```python
from build123d import *
from build123d.topology import SkipClean

# Parameters (mm, degrees)
BOSS_EXTRUDE1_DEPTH = 5
BOSS_EXTRUDE3_DEPTH = 5
BOSS_EXTRUDE4_DEPTH = 5.043608808
CIRPATTERN1_COUNT   = 3


with BuildPart() as part:
    # Sketch1 → Boss-Extrude1 (new body)
    with BuildSketch(Plane.XY):
        with BuildLine():
            ThreePointArc((0, 5), (-1.701397984, 4.701621518), (-3.199731749, 3.84209796))
            ThreePointArc((-3.199731749, 3.84209796), (-3.824264635, 3.221024682), (-4.330127019, 2.5))
            Line((-4.330127019, 2.5), (-2.165063509, 1.25))
            ThreePointArc((-2.165063509, 1.25), (-1.25, 2.165063509), (0, 2.5))
            Line((0, 2.5), (0, 5))
        make_face()
        with BuildLine():
            ThreePointArc((0, 7.5), (-1.894259298, 7.256843784), (-3.665691684, 6.54314179))
            Line((-3.665691684, 6.54314179), (-3.199731749, 3.84209796))
            ThreePointArc((-3.199731749, 3.84209796), (-1.701397984, 4.701621518), (0, 5))
            Line((0, 5), (0, 7.5))
        make_face()
        with BuildLine():
            Line((-3.199731749, 3.84209796), (-3.665691684, 6.54314179))
            ThreePointArc((-3.665691684, 6.54314179), (-5.268898566, 5.337481419), (-6.495190528, 3.75))
            Line((-6.495190528, 3.75), (-4.330127019, 2.5))
            ThreePointArc((-4.330127019, 2.5), (-3.824264635, 3.221024682), (-3.199731749, 3.84209796))
        make_face()
        with BuildLine():
            ThreePointArc((0, 14.1), (-3.800809124, 15.48736773), (-5.814119968, 18.997))
            Line((-5.814119968, 18.997), (-3.665691684, 6.54314179))
            ThreePointArc((-3.665691684, 6.54314179), (-1.894259298, 7.256843784), (0, 7.5))
            Line((0, 7.5), (0, 14.1))
        make_face()
        with BuildLine():
            ThreePointArc((0, 25.9), (-4.51263227, 23.800809124), (-5.814119968, 18.997))
            ThreePointArc((-5.814119968, 18.997), (-3.800809124, 15.48736773), (0, 14.1))
            Line((0, 14.1), (0, 16))
            ThreePointArc((0, 16), (-4, 20), (0, 24))
            Line((0, 24), (0, 25.9))
        make_face()
        with BuildLine():
            ThreePointArc((0, 2.5), (-1.25, 2.165063509), (-2.165063509, 1.25))
            Line((-2.165063509, 1.25), (0, 0))
            Line((0, 0), (0, 2.5))
        make_face()
    extrude(amount=BOSS_EXTRUDE1_DEPTH)

    # Sketch2 → Boss-Extrude3 (add)
    with BuildSketch(Plane.XY.offset(5)):
        with BuildLine():
            ThreePointArc((0, 16), (-4, 20), (0, 24))
            Line((0, 24), (0, 25.9))
            ThreePointArc((0, 25.9), (-4.51263227, 23.800809124), (-5.814119968, 18.997))
            Line((-5.814119968, 18.997), (-3.199731749, 3.84209796))
            ThreePointArc((-3.199731749, 3.84209796), (-3.824264635, 3.221024682), (-4.330127019, 2.5))
            Line((-4.330127019, 2.5), (0, 0))
            Line((0, 0), (0, 16))
        make_face()
    extrude(amount=BOSS_EXTRUDE3_DEPTH)

    # Sketch4 → Boss-Extrude4 (add)
    with BuildSketch(Plane.XY.offset(10)):
        with BuildLine():
            ThreePointArc((0, 2.5), (-1.25, 2.165063509), (-2.165063509, 1.25))
            Line((-2.165063509, 1.25), (0, 0))
            Line((0, 0), (0, 2.5))
        make_face()
        with BuildLine():
            Line((-4.330127019, 2.5), (-2.165063509, 1.25))
            ThreePointArc((-2.165063509, 1.25), (-1.25, 2.165063509), (0, 2.5))
            Line((0, 2.5), (0, 5))
            ThreePointArc((0, 5), (-1.701397984, 4.701621518), (-3.199731749, 3.84209796))
            ThreePointArc((-3.199731749, 3.84209796), (-3.824264635, 3.221024682), (-4.330127019, 2.5))
        make_face()
    extrude(amount=BOSS_EXTRUDE4_DEPTH)

    # Mirror1: part across plane


with BuildPart() as part_1:
    with SkipClean():  # the faces are left unmerged after this step: merging them gives an invalid solid
        add(part.part)
        add(part.part.mirror(Plane(origin=(0, 0, 0), x_dir=(0, 0, 1), z_dir=(1, 0, 0))))


with BuildPart() as cirpattern1_1:
    # CirPattern1: pattern copy
    add(part_1.part.rotate(Axis((0, 0, 0), (0, 0, 1)), 1 * 360 / CIRPATTERN1_COUNT))


with BuildPart() as cirpattern1_2:
    # CirPattern1: pattern copy
    add(part_1.part.rotate(Axis((0, 0, 0), (0, 0, 1)), 2 * 360 / CIRPATTERN1_COUNT))


with BuildPart() as part_2:
    add(part_1.part)

    # Combine1: union CirPattern1_2, CirPattern1_1
    add(cirpattern1_2.part)
    add(cirpattern1_1.part)

    # Sketch8 → M5 Tapped Hole1 (revolve, cut)
    with SkipClean():  # the faces are left unmerged after this step: merging them gives an invalid solid
        with BuildSketch(Plane(origin=(0, 0, 15.043608808), x_dir=(0, -1, 0), z_dir=(1, 0, 0))):
            Polygon((0, 0), (0, 15.043608808), (2.525, 15.043608808), (2.1, 14.618608808), (2.1, 0.425), (2.525, 0), align=None)
        revolve(axis=Axis((0, 0, 21.393608808), (0, 0, -1)), mode=Mode.SUBTRACT)


solid = part_2.part
```
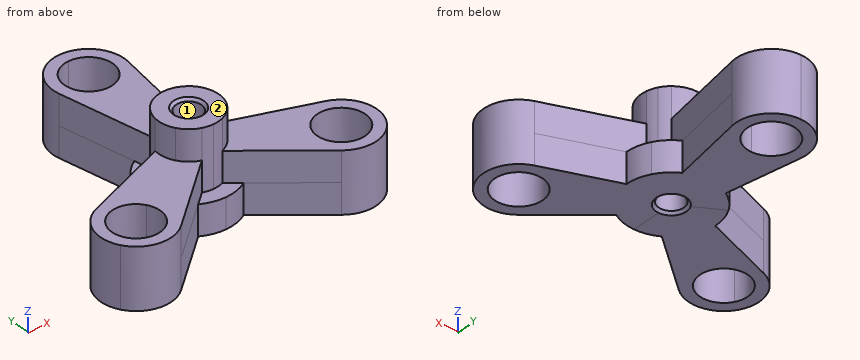
The listing builds one solid part. Answer for the finished solid, in the listing's coordinates (mm). Face numbers are marked on the shaded views. Round coordinates to 2 decimals unless told otherwise and drop trailing zeros. Write each loop counter-clockwise with the first axis right and the second up, starting at its lowest first coordinate (ties: lowest second). Pieces come first, ordered by that corner, then holes. Notation, with made-up numbers: (-25.75, -17.75) -> (28.25, -17.75) arc R7 ccw to (28.25, -12.75) -> close; hole circle Ø11 at (31, -5.5). An arc over 180 degrees is marked (long way). Use CSV: the item, a comma, the result in double quotes. Start each with the question number.
(1) Each of these flat-tipped pins is pushed along its axis until it touches: pin 1 (13 mm diameter, centred on x = -2.5, y = 18.5, fed in from +Z); pin 2 (8 mm diameter, centred on y = 16.5, z = 6.5, fed in from +X); pin 3 (2.5 mm diameter, centred on x = 0, y = 0, fed in from +Z); pin 4 (6 mm diameter, centred on y = 9.5, z = 4.5, fed in from -X). Where does it stop, or does it pass through?
(2) Section C-C on y = -10 is taken. Give the vertices of the cut face in (x, z), then the cut area to 3 significant figures.
(3) Section D-D on x = 17 is taken. Give the vertices of the cut face in (y, z), then the cut area to 3 significant figures.
(4) Section B-B on z = 1 is taken. Give the vertices of the cut face in (x, y), then the cut area to 3 significant figures.
(5) Consider L1, parallel to Y at x = 0, z = 5.5; L2, parallel to Y at x = 0, z = 4.5; L3, parallel to X at y = 0, z = 4.75. Determine where each line is inside the solid, lowest interval first. Write a range as from..to.
(6) Section A-A on y = 20 is taken. Give the vertices of the cut face in (x, z).
(7) The mould has two halves that part along Y. Classify the marked faces 1 and 2: released by +Y, released by -Y, zero draft, split by the parting line, or undercut.
A:
1,pin 1,"stops at z = 10"
1,pin 2,"stops at x = 5.9"
1,pin 3,"passes through"
1,pin 4,"stops at x = -4.69"
2,outline,"(-23.22, 0) -> (-21.32, 0) -> (-21.32, 10) -> (-23.22, 10) -> close; (-13.32, 0) -> (-8.1, 0) -> (-8.1, 10) -> (-13.32, 10) -> close; (8.1, 0) -> (13.32, 0) -> (13.32, 10) -> (8.1, 10) -> close; (21.32, 0) -> (23.22, 0) -> (23.22, 10) -> (21.32, 10) -> close"
2,area,"142 mm²"
3,outline,"(-15.89, 0) -> (-13.99, 0) -> (-13.99, 10) -> (-15.89, 10) -> close; (-6.01, 0) -> (-3.59, 0) -> (-3.59, 10) -> (-6.01, 10) -> close"
3,area,"43.2 mm²"
4,outline,"(-19.36, -4.46) arc R5.9 ccw (long way) to (-13.54, -14.53) -> (-3.83, -6.45) arc R7.5 ccw to (3.83, -6.45) -> (13.54, -14.53) arc R5.9 ccw (long way) to (19.36, -4.46) -> (7.5, -0.1) arc R7.5 ccw to (3.67, 6.54) -> (5.81, 19) arc R5.9 ccw (long way) to (-5.81, 19) -> (-3.67, 6.54) arc R7.5 ccw to (-7.5, -0.1) -> close; hole circle Ø8 at (-17.32, -10); hole circle Ø8 at (0, 20); hole circle Ø4.2 at (0, 0); hole circle Ø8 at (17.32, -10)"
4,area,"551 mm²"
5,L1,"y = -5..-2.1, 2.1..16, 24..25.9"
5,L2,"y = -7.5..-2.1, 2.1..16, 24..25.9"
5,L3,"x = -7.5..-2.1, 2.1..7.5"
6,outline,"(-5.9, 0) -> (-4, 0) -> (-4, 10) -> (-5.9, 10) -> close; (4, 0) -> (5.9, 0) -> (5.9, 10) -> (4, 10) -> close"
7,face 1,"undercut"
7,face 2,"zero draft"
